Here's how the part is built. I have some questions about the finished solid (model axes, mm). A direction names the side the tool comes from. Round coordinates to 2 decimals unless told otherwise and drop trailing zeros. Order: outer loops, then holes, each group sorted by start corner. A loop starts at its lowest first (then second) coordinate and runs counter-clockwise, first axis right, second up. Notation, with made-up numbers: M 24.5,47.25 L 81.5,47.25 A10 cw 81.5,65.25 Z; hole C -17,24.5 d8. An arc over 180 degrees is marked long. Answer as CSV lines item,"result". Start each with the question number.
```python
from build123d import *

# Parameters (mm, degrees)
BOSS_EXTRUDE1_DEPTH                                  = 3
BOSS_EXTRUDE2_DEPTH                                  = 4
REFRENTADO_PARA_TORNILLO_CON_CABEZA_PLAN_D           = 3.4
REFRENTADO_PARA_TORNILLO_CON_CABEZA_PLAN_DEPTH       = 40
REFRENTADO_PARA_TORNILLO_CON_CABEZA_PLAN_CBORE_D     = 6.5
REFRENTADO_PARA_TORNILLO_CON_CABEZA_PLAN_CBORE_DEPTH = 2
REFRENTADO_PARA_TORNILLO_CON_CABEZA_PLAN_TIP         = 1.021463052
BOSS_EXTRUDE3_START                                  = 2.5
SKETCH5_R                                            = 3
SKETCH5_R_2                                          = 1.7
BOSS_EXTRUDE3_DEPTH                                  = 2.5
BOSS_EXTRUDE4_DEPTH                                  = 3
CHAMFER1_SIZE                                        = 2.5
CHAMFER2_SIZE                                        = 1
FILLET2_R                                            = 1


with BuildPart() as part:
    # Sketch1 → Boss-Extrude1 (new body)
    with BuildSketch(Plane(origin=(0, 0, 0), x_dir=(1, 0, 0), z_dir=(0, 1, 0))):
        Polygon((0, 15), (0, 25), (-5, 25), (-5, -5), (25, -5), (25, 0), (15, 0), (15, 15), align=None)
    extrude(amount=BOSS_EXTRUDE1_DEPTH)

    # Sketch2 → Boss-Extrude2 (add)
    with BuildSketch(Plane(origin=(0, 3, 0), x_dir=(1, 0, 0), z_dir=(0, 1, 0))):
        Polygon((-5, 25), (0, 25), (0, 0), (25, 0), (25, -5), (-5, -5), align=None)
    extrude(amount=BOSS_EXTRUDE2_DEPTH)

    # Refrentado para tornillo con cabeza plana de M31
    with Locations(Plane(origin=(0, 3, 0), x_dir=(1, 0, 0), z_dir=(0, 1, 0))):
        with Locations((9, 9)):
            CounterBoreHole(REFRENTADO_PARA_TORNILLO_CON_CABEZA_PLAN_D / 2, REFRENTADO_PARA_TORNILLO_CON_CABEZA_PLAN_CBORE_D / 2, REFRENTADO_PARA_TORNILLO_CON_CABEZA_PLAN_CBORE_DEPTH, depth=REFRENTADO_PARA_TORNILLO_CON_CABEZA_PLAN_DEPTH)
            with Locations((0, 0, -(REFRENTADO_PARA_TORNILLO_CON_CABEZA_PLAN_DEPTH + REFRENTADO_PARA_TORNILLO_CON_CABEZA_PLAN_TIP / 2))):  # 118° drill point
                Cone(0, REFRENTADO_PARA_TORNILLO_CON_CABEZA_PLAN_D / 2, REFRENTADO_PARA_TORNILLO_CON_CABEZA_PLAN_TIP, mode=Mode.SUBTRACT)

    # Sketch5 → Boss-Extrude3 (add)
    with BuildSketch(Plane.XZ.offset(BOSS_EXTRUDE3_START)):
        with Locations(Location((9, -9, 0), (0, 0, 90))):
            Circle(SKETCH5_R)
        with Locations(Location((9, -9, 0), (0, 0, 90))):
            Circle(SKETCH5_R_2, mode=Mode.SUBTRACT)
    extrude(amount=-BOSS_EXTRUDE3_DEPTH)

    # Sketch6 → Boss-Extrude4 (add)
    with BuildSketch(Plane(origin=(0, 7, 0), x_dir=(1, 0, 0), z_dir=(0, 1, 0))):
        Polygon((-5, -5), (-5, 19), (3.788160363, 3.788160363), (19, -5), align=None)
    extrude(amount=BOSS_EXTRUDE4_DEPTH)

    # Chamfer1
    chamfer1_edges = [part.edges().sort_by_distance(p)[0] for p in [
        (11.394080181, 10, 0.605919819),
        (-0.605919819, 10, -11.394080181),
    ]]
    chamfer(chamfer1_edges, length=CHAMFER1_SIZE)

    # Chamfer2
    chamfer2_edges = [part.edges().sort_by_distance(p)[0] for p in [
        (15, 1.5, -15),
        (-5, 5, 5),
        (25, 7, 2.5),
        (-2.5, 7, -25),
    ]]
    chamfer(chamfer2_edges, length=CHAMFER2_SIZE)

    # Fillet2
    fillet2_edges = [part.edges().sort_by_distance(p)[0] for p in [
        (9, 0, -12),
    ]]
    fillet(fillet2_edges, radius=FILLET2_R)


solid = part.part
```
Item 1: If I drill on line 1 along Z through (x, y) = (9, -1.7); line 2 along Z through (x, y) = (9, 1.9); line 3 along X through (y, z) = (-1.5, -9), over which ranges is the centre line in solid material (lowest first)?
Item 2: Which directions (+Z, -Z, +X, -X, +Y, -Y) give clear straight access to the entire face, cutting with the end or side of a thin tool? Please do faces 4 (the cylindrical face through (6.97, -1.76, -11.21)), 5 (the flat face through (7, 1, -15)), 6 (the cylindrical face through (5.753, 2.014, -9.143)), 7 (the flat face through (5.7, 3, -7.6)), 8 (the flat face through (-2, 7, -19)).
Item 3: If we section it at A-A on z = -9: Please give me the cut outline in (x, y).
Item 4: If we section it at C-C on y = 4.5: Please give me the cut outline in (x, z).
Item 5: We'd pull the mould along Z, two halves only. Please class faces 1 (the flat face through (11.288, 7.246, 0.544)), 2 (the flat face through (3, 7, -3)), 3 (the flat face through (10.4, 1, -7.6)): pulls with the +Z half, pulls with the -Z half, needs draft (parallel to the pull), parting line crosses it, or undercut.
Item 6: If we section it at B-B on x = 9: Please give me the cut outline in (y, z).
Item 7: For P1, Ø2, axis at x = 10, y = 1, coming from the -Z side; P2, Ø3, axis at x = 3.5, z = -5.5, coming from the -Y side; P3, Ø1.5, axis at x = 19, z = 3.5, coming from the +Y side, each with a flat end and sliding along its axis, tell me the tip position at first contact or that it passes through.
Item 8: If we section it at D-D on z = -1.25: Please give me the cut outline in (x, y).
Geometry says:
1,line 1,"-12 to -10.7, -7.3 to -6"
1,line 2,"-15 to -12.25, -5.75 to 5"
1,line 3,"6 to 7.3, 10.7 to 12"
2,face 4,"-Y"
2,face 5,"-Z, +X, +Y, -Y"
2,face 6,"+Y"
2,face 7,"-Z, +X"
2,face 8,"-Z, +X, +Y"
3,outline,"M -5,0 L 5,0 A1 cw 6,-1 L 6,-2.5 L 7.3,-2.5 L 7.3,1 L 5.75,1 L 5.75,3 L 0,3 L 0,7 L 0.78,7 L 0.78,7.5 L -2.11,10 L -5,10 Z; M 10.7,-2.5 L 12,-2.5 L 12,-1 A1 cw 13,0 L 15,0 L 15,3 L 12.25,3 L 12.25,1 L 10.7,1 Z"
4,outline,"M -5,-25 L 0,-25 L 0,0 L 25,0 L 25,5 L -4,5 L -5,4 Z"
5,face 1,"pulls with the -Z half"
5,face 2,"needs draft"
5,face 3,"undercut"
6,outline,"M -2.5,-12 L -1,-12 A1 cw 0,-13 L 0,-15 L 3,-15 L 3,-12.25 L 1,-12.25 L 1,-10.7 L -2.5,-10.7 Z; M -2.5,-7.3 L 1,-7.3 L 1,-5.75 L 3,-5.75 L 3,0 L 7,0 L 7,-0.78 L 7.5,-0.78 L 10,2.11 L 10,5 L 0,5 L 0,-5 A1 cw -1,-6 L -2.5,-6 Z"
7,P1,"z = -15"
7,P2,"y = 0"
7,P3,"y = 7"
8,outline,"M -5,0 L 15,0 L 15,3 L 0,3 L 0,7 L 8.18,7 L 8.18,7.5 L 3.18,10 L -5,10 Z"
